from build123d import *

# Parameters (mm, degrees)
SKETCH1_W           = 40
SKETCH1_H           = 40
BOSS_EXTRUDE1_DEPTH = 290
SKETCH2_R           = 2.3
CUT_EXTRUDE1_DEPTH  = 290
CUT_EXTRUDE2_DEPTH  = 290


with BuildPart() as part:
    # Sketch1 → Boss-Extrude1 (new body)
    with BuildSketch(Plane.XY):
        with Locations((20, 20)):
            Rectangle(SKETCH1_W, SKETCH1_H)
    extrude(amount=-BOSS_EXTRUDE1_DEPTH)

    # Sketch2 → Cut-Extrude1 (cut)
    with BuildSketch(Plane.XY):
        with Locations((10, 30)):
            Circle(SKETCH2_R)
        with Locations((30, 30)):
            Circle(SKETCH2_R)
        with Locations((30, 10)):
            Circle(SKETCH2_R)
        with Locations((10, 10)):
            Circle(SKETCH2_R)
        Polygon((6.605, 38.815), (6.605, 38.2), (4.5, 38.2), (4.5, 36.772792206), (7.372792206, 33.9), (12.627207794, 33.9), (15.5, 36.772792206), (15.5, 38.2), (13.395, 38.2), (13.395, 38.815), (14.58, 40), (5.42, 40), align=None)
        Polygon((26.605, 38.815), (25.42, 40), (34.58, 40), (33.395, 38.815), (33.395, 38.2), (35.5, 38.2), (35.5, 36.772792206), (32.627207794, 33.9), (27.372792206, 33.9), (24.5, 36.772792206), (24.5, 38.2), (26.605, 38.2), align=None)
        Polygon((26.605, 1.8), (26.605, 1.185), (25.42, 0), (34.58, 0), (33.395, 1.185), (33.395, 1.8), (35.5, 1.8), (35.5, 3.227207794), (32.627207794, 6.1), (27.372792206, 6.1), (24.5, 3.227207794), (24.5, 1.8), align=None)
        Polygon((13.395, 1.185), (14.58, 0), (5.42, 0), (6.605, 1.185), (6.605, 1.8), (4.5, 1.8), (4.5, 3.227207794), (7.372792206, 6.1), (12.627207794, 6.1), (15.5, 3.227207794), (15.5, 1.8), (13.395, 1.8), align=None)
        Polygon((1.8, 13.395), (1.185, 13.395), (0, 14.58), (0, 5.42), (1.185, 6.605), (1.8, 6.605), (1.8, 4.5), (3.227207794, 4.5), (6.1, 7.372792206), (6.1, 12.627207794), (3.227207794, 15.5), (1.8, 15.5), align=None)
        Polygon((1.185, 26.605), (0, 25.42), (0, 34.58), (1.185, 33.395), (1.8, 33.395), (1.8, 35.5), (3.227207794, 35.5), (6.1, 32.627207794), (6.1, 27.372792206), (3.227207794, 24.5), (1.8, 24.5), (1.8, 26.605), align=None)
        Polygon((38.2, 15.5), (38.2, 13.395), (38.815, 13.395), (40, 14.58), (40, 5.42), (38.815, 6.605), (38.2, 6.605), (38.2, 4.5), (36.772792206, 4.5), (33.9, 7.372792206), (33.9, 12.627207794), (36.772792206, 15.5), align=None)
        Polygon((38.2, 26.605), (38.815, 26.605), (40, 25.42), (40, 34.58), (38.815, 33.395), (38.2, 33.395), (38.2, 35.5), (36.772792206, 35.5), (33.9, 32.627207794), (33.9, 27.372792206), (36.772792206, 24.5), (38.2, 24.5), align=None)
    extrude(amount=-CUT_EXTRUDE1_DEPTH, mode=Mode.SUBTRACT)

    # Sketch3 → Cut-Extrude2 (cut)
    with BuildSketch(Plane.XY):
        Polygon((17.3, 38.2), (22.7, 38.2), (22.7, 36.027207794), (26.1, 32.627207794), (26.1, 27.372792206), (27.372792206, 26.1), (32.627207794, 26.1), (36.027207794, 22.7), (38.2, 22.7), (38.2, 17.3), (36.027207794, 17.3), (32.627207794, 13.9), (27.372792206, 13.9), (26.1, 12.627207794), (26.1, 7.372792206), (22.7, 3.972792206), (22.7, 1.8), (17.3, 1.8), (17.3, 3.972792206), (13.9, 7.372792206), (13.9, 12.627207794), (12.627207794, 13.9), (7.372792206, 13.9), (3.972792206, 17.3), (1.8, 17.3), (1.8, 22.7), (3.972792206, 22.7), (7.372792206, 26.1), (12.627207794, 26.1), (13.9, 27.372792206), (13.9, 32.627207794), (17.3, 36.027207794), align=None)
    extrude(amount=-CUT_EXTRUDE2_DEPTH, mode=Mode.SUBTRACT)


solid = part.part
Geometry: final body of the model. Coordinates: model frame, mm. A direction names the side the tool comes from. Give positions to 0.01 mm unless a question says otherwise; leave off trailing zeros. Return JSON: item names as keys, results as strings. Group by question number.
1) Set-up query: faces 4 (the flat face through (33.9, 30, -143)), 5 (the flat face through (10, 6.1, -143)), 6 (the flat face through (38.2, 20, -143)). Return all of +Z, -Z, +X, -X, +Y, -Y with unobstructed straight access to the full face (end or side cutting, diameter ignored); none if empty.
2) Mould query, pull axis X, two halves, no side actions, for faces 1 (the flat face through (26.1, 30, -143)), 2 (the flat face through (37, 0, -143)), 3 (the flat face through (0, 37, -143)). Classes: released by +X, released by -X, zero draft, split by the parting line, or undercut.
3) Line query: line 1 (X direction, y = 37, z = -136); line 2 (Y direction, x = 10, z = -79). Output: solid intervals per line, ascending.
4) Section A-A on z = -171. State how many separate pieces and enclosed holes the cut face has, plus the area to 3 significant figures.
5) First-contact query: P1, Ø8, axis at x = 17, y = 8.5, coming from the +Z side; P2, Ø4, axis at x = 30, y = 10, coming from the -Z side; P3, Ø1.1, axis at x = 6, z = -106, coming from the -Y side; P4, Ø2, axis at y = 33.5, z = -98, coming from the +X side. Flat tips, straight axial feed; report the tip coordinate or a pass-through.
Filled in:
{
 "1": {"face 4": "+Z, -Z, +X", "face 5": "+Z, -Z, -Y", "face 6": "+Z, -Z"},
 "2": {"face 1": "undercut", "face 2": "zero draft", "face 3": "released by -X"},
 "3": {"line 1": "x = 0 to 4.5, 15.5 to 17.3, 22.7 to 24.5, 35.5 to 40", "line 2": "y = 6.1 to 7.7, 12.3 to 13.9, 26.1 to 27.7, 32.3 to 33.9"},
 "4": {"separate pieces": "1", "enclosed holes": "5", "area": "475 mm^2"},
 "5": {"P1": "stops at z = 0", "P2": "passes through", "P3": "stops at y = 0.03", "P4": "stops at x = 39.92"}
}
